Here's how the part is built. I have some questions about the finished solid (model axes, mm). A direction names the side the tool comes from. Coordinates: 2 decimals unless noted, no trailing zeros. Order: outer loops, then holes, each group sorted by start corner. A loop starts at its lowest first (then second) coordinate and runs counter-clockwise, first axis right, second up. Notation, with made-up numbers: (59, 31.25) - (114, 31.25) arc R10 ccw to (114, 47.25) - close; hole circle Ø1 at (29.5, 55.5). An arc over 180 degrees is marked (long way). Use CSV: the item, a comma, the result in double quotes. Start each with the question number.
from build123d import *

# Parameters (mm, degrees)
F0_W     = 137
F0_H     = 134
F1_DEPTH = 1
F2_W     = 137
F2_H     = 1
F3_DEPTH = 35
F4_R     = 1.5
F4_W     = 1.5
F4_H     = 20
F5_DEPTH = 136.001
F6_R     = 0.5


with BuildPart() as f1:
    # F0 (on Top) → F1 (new body)
    with BuildSketch(Plane.XY):
        Rectangle(F0_W, F0_H)
    extrude(amount=F1_DEPTH)

    # F2 (on face) → F3 (join)
    with BuildSketch(Plane.XY.offset(1)):
        with Locations((0, -67.5)):
            Rectangle(F2_W, F2_H)
        with Locations((0, 67.5)):
            Rectangle(F2_W, F2_H)
    extrude(amount=-F3_DEPTH)

    # F4 (on face) → F5 (cut, through all)
    with BuildSketch(Plane.XZ.offset(68)):
        with Locations((-54, -27)):
            Circle(F4_R)
        with Locations((54, -27)):
            Circle(F4_R)
        with Locations((-25, -16)):
            Rectangle(F4_W, F4_H)
        with Locations((-20, -16)):
            Rectangle(F4_W, F4_H)
        with Locations((-15, -16)):
            Rectangle(F4_W, F4_H)
        with Locations((-10, -16)):
            Rectangle(F4_W, F4_H)
        with Locations((-5, -16)):
            Rectangle(F4_W, F4_H)
        with Locations((0, -16)):
            Rectangle(F4_W, F4_H)
        with Locations((5, -16)):
            Rectangle(F4_W, F4_H)
        with Locations((10, -16)):
            Rectangle(F4_W, F4_H)
        with Locations((15, -16)):
            Rectangle(F4_W, F4_H)
        with Locations((20, -16)):
            Rectangle(F4_W, F4_H)
        with Locations((25, -16)):
            Rectangle(F4_W, F4_H)
    extrude(amount=-F5_DEPTH, mode=Mode.SUBTRACT)

    # F6
    f6_edges = [f1.edges().sort_by_distance(p)[0] for p in [
        (0, -68, 1),
        (0, 68, 1),
        (0, -67, 0),
        (0, 67, 0),
    ]]
    fillet(f6_edges, radius=F6_R)


solid = f1.part
Item 1: For faces 1 (the flat face through (-1, -67, -17)), 2 (the cylindrical face through (-54.195, 67.493, -25.513)), which set-ups out of +Z, -Z, +X, -X, +Y, -Y let a thin tool reach every point of the face, with its end or its side?
Item 2: Suppose I cut it at C-C on z = -12. State how many separate pieces and enclosed holes the cut face has, then the cut area to 3 significant figures.
Item 3: Suppose I cut it at D-D on y = 46.5. Write out the boundary of the cut face in (x, z).
Item 4: We'd pull the mould along Y, two halves only. Please class faces 3 (the flat face through (-1, -68, -17)), 4 (the cylindrical face through (54.806, -67.507, -25.735)), 5 (the flat face through (-1, 67, -17)), 6 (the flat face through (-1, 1, 0)): released by +Y, released by -Y, zero draft, split by the parting line, or undercut.
Item 5: Please list where these lines run through material, in increasing order: line 1 along Z through (x, y) = (-54, -67.3); line 2 along Y through (x, z) = (24, -9.5); line 3 along Z through (x, y) = (-55.5, 56.5). Write a range as from..to.
Item 6: Suppose I cut it at B-B on x = 28.5. Write out the boundary of the cut face in (y, z).
Item 7: For pin 1 Ø4 at (x, y) = (15.5, -17.5) entering from -Z, with a flat end and sliding along its axis, tell me the tip position at first contact or that it passes through.
Item 8: Suppose I cut it at A-A on z = -31. Write out the boundary of the cut face in (x, y), then the cut area to 3 significant figures.
Here are the results:
1,face 1,"-Z, +X, -X"
1,face 2,"+Y, -Y"
2,separate pieces,"24"
2,enclosed holes,"0"
2,area,"241 mm^2"
3,outline,"(-68.5, 0) - (68.5, 0) - (68.5, 1) - (-68.5, 1) - close"
4,face 3,"released by -Y"
4,face 4,"zero draft"
4,face 5,"undercut"
4,face 6,"undercut"
5,line 1,"-34..-28.5, -25.5..1"
5,line 2,"-68..-67, 67..68"
5,line 3,"0..1"
6,outline,"(-68, -34) - (-67, -34) - (-67, -0.5) arc R0.5 cw to (-66.5, 0) - (66.5, 0) arc R0.5 cw to (67, -0.5) - (67, -34) - (68, -34) - (68, 0.5) arc R0.5 ccw to (67.5, 1) - (-67.5, 1) arc R0.5 ccw to (-68, 0.5) - close"
7,pin 1,"z = 0"
8,outline,"(-68.5, -68) - (68.5, -68) - (68.5, -67) - (-68.5, -67) - close; (-68.5, 67) - (68.5, 67) - (68.5, 68) - (-68.5, 68) - close"
8,area,"274 mm^2"
